from build123d import *

# Parameters (mm, degrees)
SKETCH2_R          = 1.5
CUT_EXTRUDE1_DEPTH = 10


with BuildPart() as part:
    # Sketch1 → Revolve1 (revolve)
    with BuildSketch(Plane.XY, mode=Mode.PRIVATE) as revolve1_sk:
        Polygon((-24.5, 0), (-24.5, 3), (-9.5, 3), (-9.5, 10), (-4.5, 10), (-4.5, 20), (26.5, 20), (26.5, 0), align=None)
    revolve(revolve1_sk.sketch.rotate(Axis((-28.153846154, 0, 0), (1, 0, 0)), 90), axis=Axis((-28.153846154, 0, 0), (1, 0, 0)))

    # Sketch2 → Cut-Extrude1 (cut)
    with BuildSketch(Plane.ZY.offset(4.5)):
        with Locations((15, 0)):
            Circle(SKETCH2_R)
        with Locations((-7.5, -12.990381057)):
            Circle(SKETCH2_R)
        with Locations((-7.5, 12.990381057)):
            Circle(SKETCH2_R)
    extrude(amount=-CUT_EXTRUDE1_DEPTH, mode=Mode.SUBTRACT)


solid = part.part
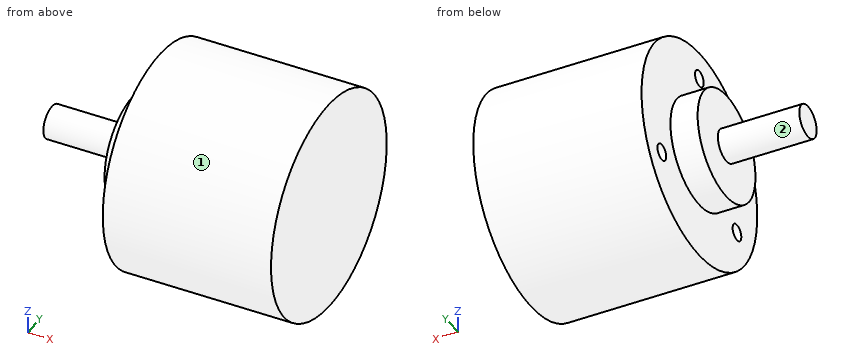
The model under review builds one solid part; all positions refer to its coordinate system, in mm. Face numbers are marked on the shaded views. A direction names the side the tool comes from. Coordinates: 2 decimals unless noted, no trailing zeros. Loops run counter-clockwise (first coordinate to the right, second up) from the corner with the lowest first, then second, coordinate; pieces in that order, holes last.
(1) Consider section B-B, the plane z = 0. Give the boundary of the cut face in (x, y), plus the area to 3 significant figures.
Determined:
outline: (-24.5, -3) - (-9.5, -3) - (-9.5, -10) - (-4.5, -10) - (-4.5, -20) - (26.5, -20) - (26.5, 20) - (-4.5, 20) - (-4.5, 10) - (-9.5, 10) - (-9.5, 3) - (-24.5, 3) - close
area: 1,430 mm2
(2) Consider section C-C, the plane x = 23.5. Give the boundary of the cut face in (y, z), plus the area to 3 significant figures.
Determined:
outline: circle Ø40 at (0, 0)
area: 1,260 mm2
(3) Consider section A-A, the plane y = 0. Give the boundary of the cut face in (x, z).
Determined:
outline: (-24.5, -3) - (-9.5, -3) - (-9.5, -10) - (-4.5, -10) - (-4.5, -20) - (26.5, -20) - (26.5, 20) - (-4.5, 20) - (-4.5, 16.5) - (5.5, 16.5) - (5.5, 13.5) - (-4.5, 13.5) - (-4.5, 10) - (-9.5, 10) - (-9.5, 3) - (-24.5, 3) - close
(4) Consider section D-D, the plane z = 15. Give the boundary of the cut face in (x, y).
Determined:
outline: (-4.5, -13.23) - (26.5, -13.23) - (26.5, 13.23) - (-4.5, 13.23) - (-4.5, 1.5) - (5.5, 1.5) - (5.5, -1.5) - (-4.5, -1.5) - close
(5) Tool access review of the marked faces 1 and 2: name each direction out of +Z, -Z, +X, -X, +Y, -Y from which nothing blocks a thin tool from reaching the whole face with its end or side.
Determined:
face 1: +X, -X
face 2: -X
(6) Insertion check: P1, Ø12, axis at y = -13, z = -14, coming from the -X side; P2, Ø4, axis at x = 14, y = 10, coming from the -Z side; P3, Ø4, axis at x = 16.5, y = 7.5, coming from the +Z side; P4, Ø10, axis at x = -16, y = -11, coming from the +Z side. Each pin has a flat end and moves straight along its axis. Give the tip position at first contact, or say it passes through.
Determined:
P1: stops at x = -4.5
P2: stops at z = -18.33
P3: stops at z = 19.23
P4: passes through
(7) Wall thickness on L1, parallel to Y at x = 2.25, z = -7.5; L2, parallel to Y at x = 0, z = -7 (3 decimals); L3, parallel to X at y = -6.5, z = 3.5: over which ranges is each line inside the solid? List them lowest first.
Determined:
L1: y = -18.54 to -14.49, -11.49 to 11.49, 14.49 to 18.54
L2: y = -18.735 to -14.405, -11.576 to 11.576, 14.405 to 18.735
L3: x = -9.5 to 26.5
